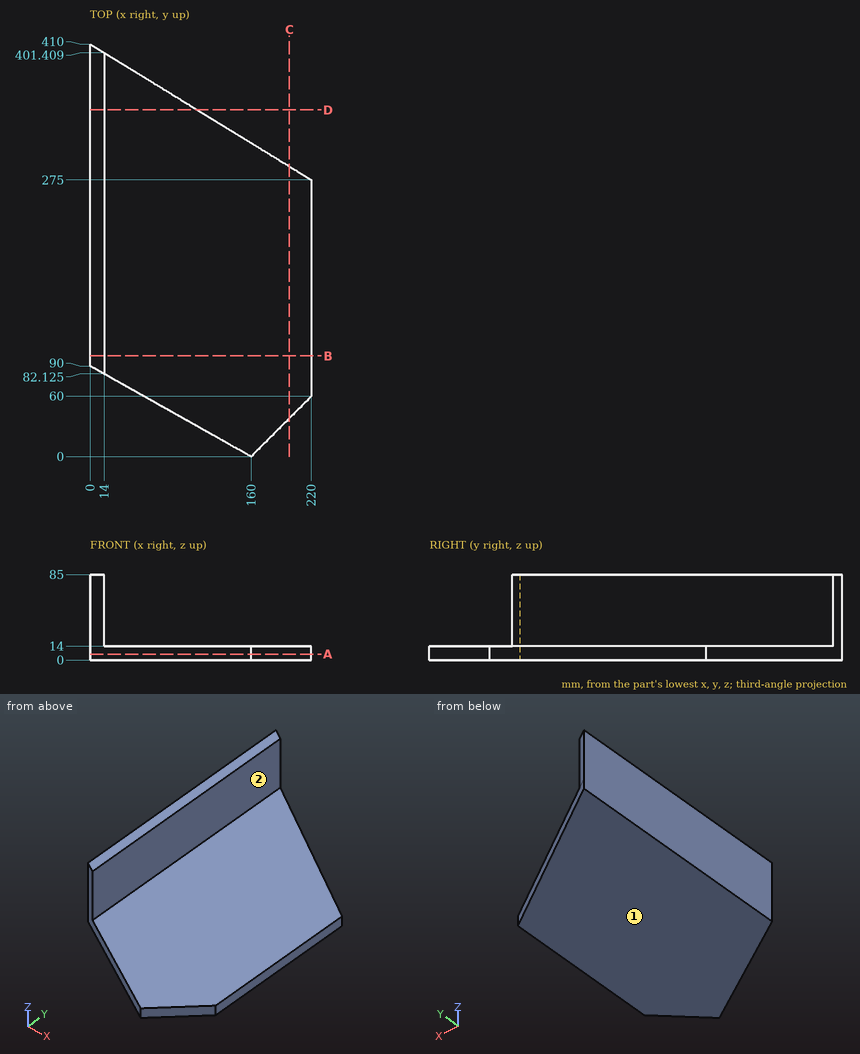
Input: dimensioned drawing with shaded views. Units: mm. Origin: part minimum x, y, z. A direction names the side the tool comes from. Give positions to 0.01 mm unless a question says otherwise; leave off trailing zeros. Loops run counter-clockwise (first coordinate to the right, second up) from the corner with the lowest first, then second, coordinate; pieces in that order, holes last. Notation, with made-up numbers: (10.25, -2.5) -> (35.25, -2.5) arc R6 ccw to (35.25, 1.5) -> close; hole circle Ø2 at (-5.5, -20.75). An arc over 180 degrees is marked (long way). Use a Markdown table: item, result.
Q1. Ray query, probe 1 along Z at (x, y) = (196.5, 268). Return the intervals inside material, ascending. Write a range as from..to.
Entries:
| item | result |
|---|---|
| probe 1 | z = 0..14 |
Q2. First-contact query: P1, Ø1.5, axis at x = 195, y = 89, coming from the +Z side; P2, Ø5, axis at y = 216.5, z = 50, coming from the +X side. Flat tips, straight axial feed; report the tip coordinate or a pass-through.
Entries:
| item | result |
|---|---|
| P1 | stops at z = 14 |
| P2 | stops at x = 14 |
Q3. Access query for the marked faces 1 and 2. Directions: +Z, -Z, +X, -X, +Y, -Y. A direction counts if a zero-diameter tool reaches every point of the face in a straight line with its end or side. Return the directions, or none.
Entries:
| item | result |
|---|---|
| face 1 | -Z, +X, -X, +Y, -Y |
| face 2 | +Z, +X, +Y, -Y |
Q4. Section query B-B, the plane y = 100. Return the cut outline in (x, z).
Entries:
| item | result |
|---|---|
| outline | (0, 0) -> (220, 0) -> (220, 14) -> (14, 14) -> (14, 85) -> (0, 85) -> close |
Q5. Section query D-D, the plane y = 344.5. Return the cut outline in (x, z).
Entries:
| item | result |
|---|---|
| outline | (0, 0) -> (106.74, 0) -> (106.74, 14) -> (14, 14) -> (14, 85) -> (0, 85) -> close |
Q6. Section query A-A, the plane z = 6. Return the cut outline in (x, y).
Entries:
| item | result |
|---|---|
| outline | (0, 90) -> (160, 0) -> (220, 60) -> (220, 275) -> (0, 410) -> close |
Q7. Section query C-C, the plane x = 198. Return the cut outline in (y, z).
Entries:
| item | result |
|---|---|
| outline | (38, 0) -> (288.5, 0) -> (288.5, 14) -> (38, 14) -> close |
